Design review of the part built by this model. Coordinates are the model's own, in mm. Face numbers are marked on the shaded views. A direction names the side the tool comes from. Coordinates: 2 decimals unless noted, no trailing zeros. Loops run counter-clockwise (first coordinate to the right, second up) from the corner with the lowest first, then second, coordinate; pieces in that order, holes last. Notation, with made-up numbers: M 62.5,-3 L 80.5,-3 A18 ccw 80.5,3 Z; hole C -9.75,-39.5 d1. An arc over 180 degrees is marked long. Answer as a JSON object with one key per item and string values. Group by question number.
1. Machinability: for the marked faces 1 and 2, which of the approach directions +Z, -Z, +X, -X, +Y, -Y give a long, thin tool a straight path to every point of the face, cutting with its end or side? Answer none if there is none.
2. Consider section D-D (z = -14). State the section outline as (x, y) points.
3. To check wall thickness, follow probe 1 along X at (y, z) = (-7, 0); probe 2 along Y at (x, z) = (99.5, 0). State the ranges of each line that lie inside material, in increasing order.
4. Consider section B-B (y = -73.5). State the section outline as (x, z) points, then the cut area to 3 significant figures.
5. Insertion check: pin 1 (13 mm diameter, centred on x = -93.5, z = 0, fed in from -Y); pin 2 (6 mm diameter, centred on x = -95, y = -26.5, fed in from +Z); pin 3 (13 mm diameter, centred on x = -98.5, y = -37.5, fed in from -Z). Each pin has a flat end and moves straight along its axis. Give the tip position at first contact, or say it passes through.
6. Consider section C-C (y = -20.5). State the section outline as (x, z) points.
7. Consider section A-A (x = 0). State the section outline as (y, z) points, then the cut area to 3 significant figures.
8. Draft analysis for pull direction Z (two halves, no side actions). For the marked faces 3, 4 and 5, state which applies: +Z half, -Z half, draft (parallel to the pull), parting line (faces both ways), or undercut.
from build123d import *

# Parameters (mm, degrees)
SKETCH1_R                = 102
SKETCH1_R_2              = 90
BOSS_EXTRUDE1_DEPTH      = 25.4
BOSS_EXTRUDE4_DEPTH      = 12
SKETCH14_W               = 3.541917671
SKETCH14_H               = 50
CUT_EXTRUDE2_DEPTH       = 25.4
SKETCH8_W                = 60
SKETCH8_H                = 84.7705
BOSS_EXTRUDE5_DEPTH      = 12
M8_CLEARANCE_HOLE1_D     = 10
M8_CLEARANCE_HOLE1_DEPTH = 12


with BuildPart() as part:
    # Sketch1 → Boss-Extrude1 (new body)
    with BuildSketch(Plane(origin=(0, 0, 0), x_dir=(1, 0, 0), z_dir=(0, 1, 0))):
        Circle(SKETCH1_R)
        Circle(SKETCH1_R_2, mode=Mode.SUBTRACT)
    extrude(amount=-BOSS_EXTRUDE1_DEPTH)

    # Sketch7 → Boss-Extrude4 (add)
    with BuildSketch(Plane(origin=(-90, 0, 0), x_dir=(0, 0, -1), z_dir=(1, 0, 0))):
        Polygon((-25, -25.4), (-25, -81.8336), (25, -81.8336), (25, -25.4), (25, 0), (-25, 0), align=None)
    extrude(amount=-BOSS_EXTRUDE4_DEPTH)

    # Sketch14 → Cut-Extrude2 (cut)
    with BuildSketch(Plane.XZ.offset(25.4)):
        with Locations((-88.229041165, 0)):
            Rectangle(SKETCH14_W, SKETCH14_H)
    extrude(amount=-CUT_EXTRUDE2_DEPTH, mode=Mode.SUBTRACT)

    # Sketch8 → Boss-Extrude5 (add)
    with BuildSketch(Plane.ZY.offset(-90)):
        with Locations((0, -42.38525)):
            Rectangle(SKETCH8_W, SKETCH8_H)
    extrude(amount=-BOSS_EXTRUDE5_DEPTH)

    # M8 Clearance Hole1
    with Locations(Plane.ZY.offset(-90)):
        with Locations((0, -59.7705)):
            Hole(M8_CLEARANCE_HOLE1_D / 2, depth=M8_CLEARANCE_HOLE1_DEPTH)


solid = part.part
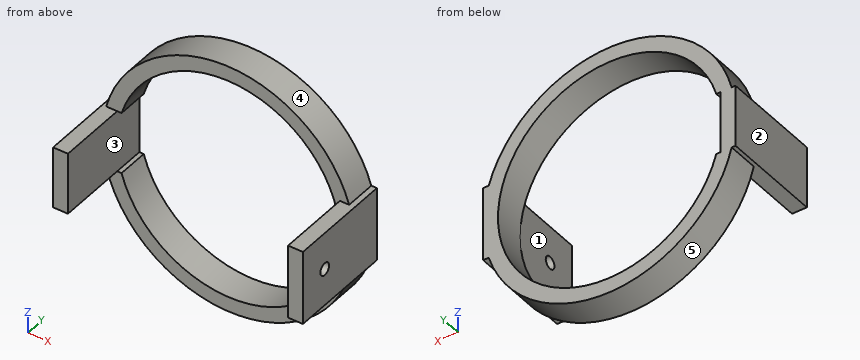
Findings below:
{
 "1": {"face 1": "+Z, -Z, -Y", "face 2": "+Z, -Z, -X, +Y, -Y"},
 "2": {"outline": "M -102,-81.83 L -90,-81.83 L -90,0 L -102,0 Z; M 88.9,-25.4 L 90,-25.4 L 90,-84.77 L 102,-84.77 L 102,0 L 88.9,0 Z"},
 "3": {"probe 1": "x = -102 to -90, 90 to 102", "probe 2": "y = -84.77 to -64.77, -54.77 to 0"},
 "4": {"outline": "M -102,-25 L -90,-25 L -90,25 L -102,25 Z; M 90,-30 L 102,-30 L 102,30 L 90,30 Z", "area": "1,320 mm^2"},
 "5": {"pin 1": "stops at y = -81.83", "pin 2": "stops at z = 43.61", "pin 3": "stops at z = -25"},
 "6": {"outline": "M -102,-25 L -98.89,-25 A102 ccw 97.49,-30 L 102,-30 L 102,30 L 97.49,30 A102 ccw -98.89,25 L -102,25 Z; hole M -90,-25 L -86.46,-25 A90 ccw long -86.46,25 L -90,25 Z"},
 "7": {"outline": "M -25.4,-102 L 0,-102 L 0,-90 L -25.4,-90 Z; M -25.4,90 L 0,90 L 0,102 L -25.4,102 Z", "area": "610 mm^2"},
 "8": {"face 3": "undercut", "face 4": "+Z half", "face 5": "-Z half"}
}
